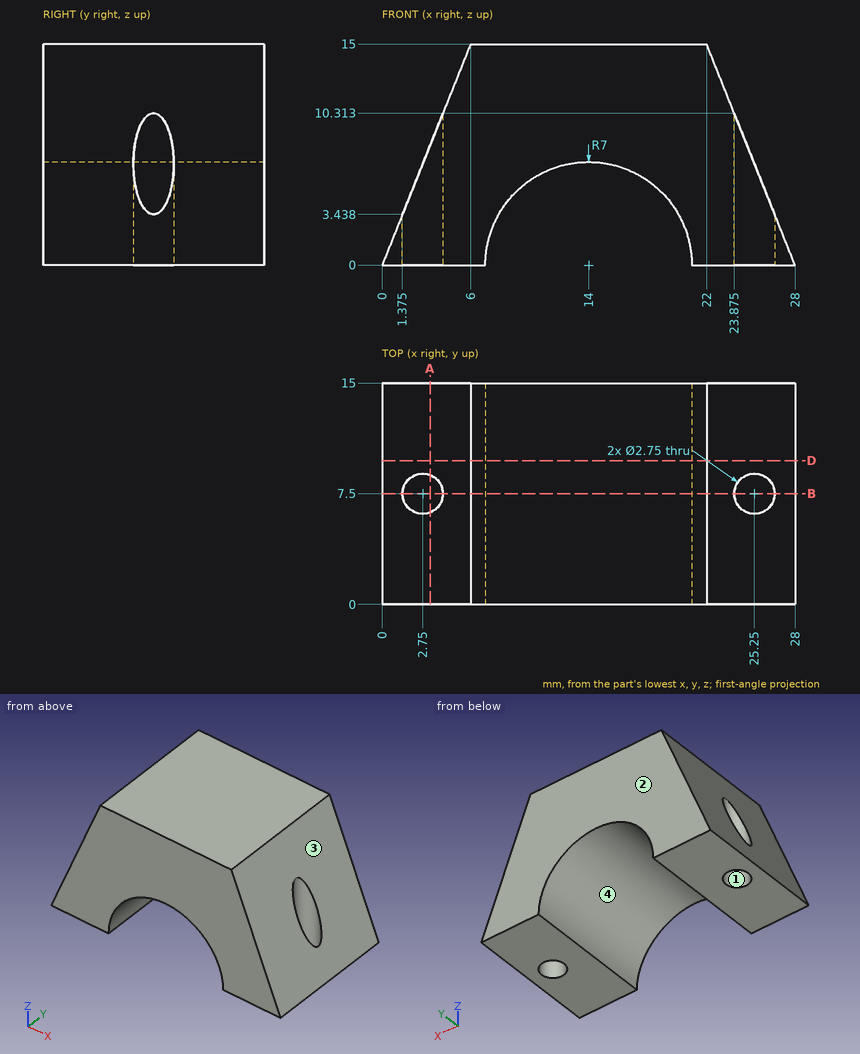
Check sheet for the drawn part. Datum: minimum x, y, z corner. Units: mm. Round coordinates to 2 decimals unless told otherwise and drop trailing zeros. Order: outer loops, then holes, each group sorted by start corner. A loop starts at its lowest first (then second) coordinate and runs counter-clockwise, first axis right, second up. Notation, with made-up numbers: M -16,41 L 29,41 A31 ccw 29,69 Z; hole C 56,88.5 d7. An arc over 180 degrees is marked long. Write each question's results on one line, items separated by ' | '. Start each with the question number.
1. Cross-section at A-A on x = 3.25. Record the boundary of the cut face in (y, z) (1 decimal), plus the area to 3 significant figures.
2. Draft check along X on the marked faces 1, 2, 3 and 4. Enter one of: pulls with the +X half, pulls with the -X half, needs draft (parallel to the pull), parting line crosses it, or undercut.
3. Go/stop test with flat-tipped pins: P1, Ø8, axis at y = 9, z = 9.5, coming from the +X side; P2, Ø3, axis at x = 18, z = 9, coming from the -Y side. Record where each tip stops, or that it passes through.
4. Cross-section at D-D on y = 9.75. Record the boundary of the cut face in (x, z).
5. Material ranges on L1, parallel to Y at x = 2.75, z = 6 (1 decimal); L2, parallel to X at y = 7.5, z = 3 (1 decimal); L3, parallel to X at y = 1.75, z = 6 (1 decimal), recorded low to high. Write a range as from..to.
6. Cross-section at B-B on y = 7.5. Record the boundary of the cut face in (x, z) (1 decimal).
Resolved:
1) outline: M 0,0 L 6.2,0 L 6.2,8.1 L 0,8.1 Z; M 8.8,0 L 15,0 L 15,8.1 L 8.8,8.1 Z | area: 101 mm2
2) face 1: undercut | face 2: needs draft | face 3: pulls with the +X half | face 4: undercut
3) P1: x = 25.8 | P2: y = 0
4) outline: M 0,0 L 7,0 A7 cw 21,0 L 28,0 L 22,15 L 6,15 Z
5) L1: 0..6.1, 8.9..15 | L2: 1.2..1.4, 4.1..7.7, 20.3..23.9, 26.6..26.8 | L3: 2.4..10.4, 17.6..25.6
6) outline: M 0,0 L 1.4,0 L 1.4,3.4 Z; M 4.1,0 L 7,0 A7 cw 21,0 L 23.9,0 L 23.9,10.3 L 22,15 L 6,15 L 4.1,10.3 Z; M 26.6,0 L 28,0 L 26.6,3.4 Z
